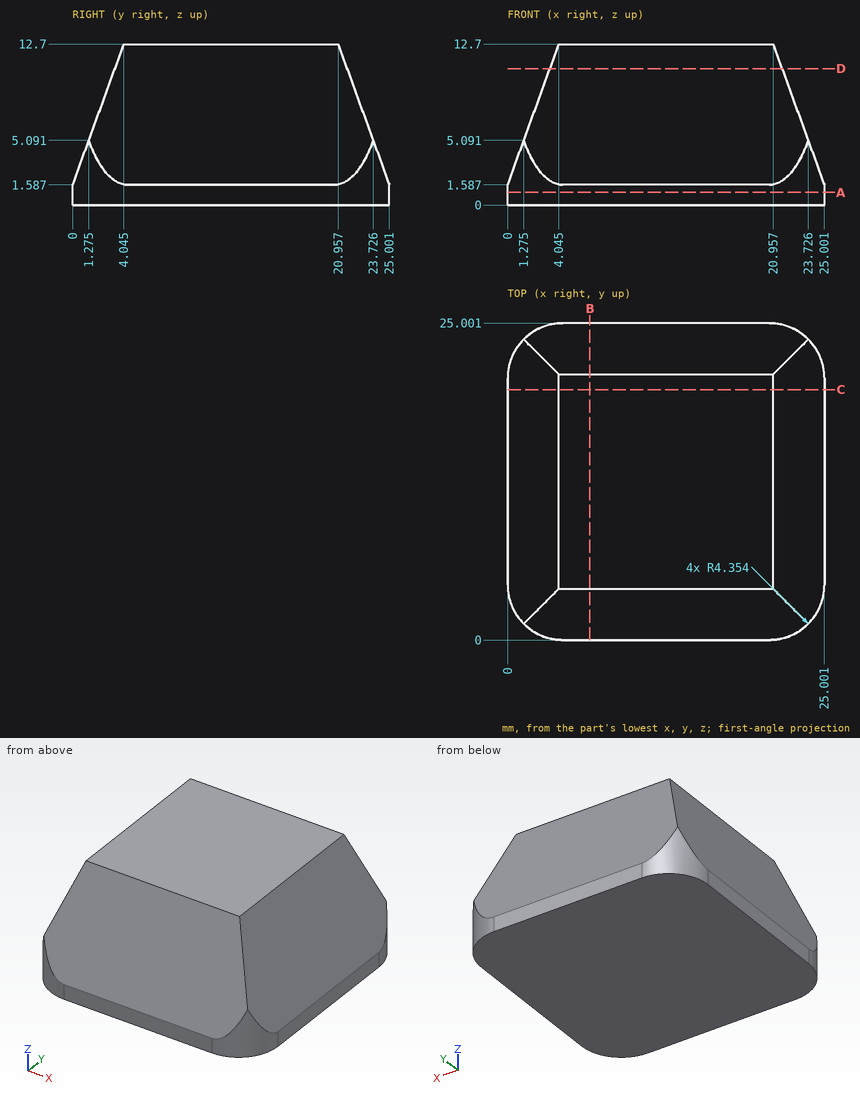
Study the drawing (mm; zero at the part's minimum x, y, z) and answer. Round coordinates to 2 decimals unless told otherwise and drop trailing zeros. Loops run counter-clockwise (first coordinate to the right, second up) from the corner with the lowest first, then second, coordinate; pieces in that order, holes last. Notation, with made-up numbers: (86, -37.75) - (110, -37.75) arc R35 ccw to (110, -4.75) - close; hole circle Ø9 at (7.5, 43.5). An arc over 180 degrees is marked (long way). Use one line per item in the form item = value. Start each with the question number.
1. The part is cut by section A-A on z = 1. Determine the outline of the cut face in (x, y) (1 decimal).
2. Given pin 1 Ø5 at (x, z) = (13, 8) entering from -Y (1 decimal); pin 2 Ø3 at (y, z) = (9.5, 2) entering from +X, each flat-ended and moving along its own axis, determine where each tip first touches the part or whether it passes through.
3. The part is cut by section D-D on z = 10.75. Determine the outline of the cut face in (x, y) (1 decimal), then the cut area to 3 significant figures.
4. The part is cut by section B-B on x = 6.5. Determine the outline of the cut face in (y, z) (1 decimal), then the cut area to 3 significant figures.
5. Consider line 1 (X direction, y = 15, z = 8.5) (1 decimal); line 2 (X direction, y = 2.75, z = 8.75) (1 decimal); line 3 (Y direction, x = 21.5, z = 5). Determine where each line is inside the solid, lowest interval first. Write a range as [from, to].
Geometry check:
q1.outline = (0, 4.4) arc R4.4 ccw to (4.4, 0) - (20.6, 0) arc R4.4 ccw to (25, 4.4) - (25, 20.6) arc R4.4 ccw to (20.6, 25) - (4.4, 25) arc R4.4 ccw to (0, 20.6) - close
q2.pin_1 = 1.4
q2.pin_2 = 25
q3.outline = (3.3, 3.3) - (21.7, 3.3) - (21.7, 21.7) - (3.3, 21.7) - close
q3.area = 336 mm^2
q4.outline = (0, 0) - (25, 0) - (25, 1.6) - (21, 12.7) - (4, 12.7) - (0, 1.6) - close
q4.area = 273 mm^2
q5.line_1 = [2.5, 22.5]
q5.line_2 = [2.6, 22.4]
q5.line_3 = [1.24, 23.76]
